Design review of the part shown in the three views and the two pictorial views. Dimensions are in mm from the part's minimum x, y and z. A direction names the side the tool comes from. Round coordinates to 2 decimals unless told otherwise and drop trailing zeros. Loops run counter-clockwise (first coordinate to the right, second up) from the corner with the lowest first, then second, coordinate; pieces in that order, holes last.
1. To check wall thickness, follow line 1 along Z through (x, y) = (34, 12.7); line 2 along X through (y, z) = (11.5, 7.5); line 3 along X through (y, z) = (11.25, 10.5). State the ranges of each line that lie inside material, in increasing order.
2. Draft analysis for pull direction X (two halves, no side actions). For the marked faces 4, 5 and 6, state which applies: released by +X, released by -X, zero draft, split by the parting line, or undercut.
3. Clearance check with flat-ended pins moving along their axes: pin 1 Ø12 at (y, z) = (12, 31.5) entering from -X; pin 2 Ø12 at (x, y) = (33, 3) entering from +Z; pin 3 Ø2 at (x, y) = (57.5, 4) entering from +Z. State where each tip first meets the part, or that it passes through.
4. Consider section D-D on x = 36. State the section outline as (y, z) points.
5. Consider section A-A on y = 13.5. State the section outline as (x, z) points, then the cut area to 3 significant figures.
6. Consider section C-C on x = 7.5. State the section outline as (y, z) points, then the cut area to 3 significant figures.
7. Tool access review of the marked faces 1, 2 and 3: name each direction out of +Z, -Z, +X, -X, +Y, -Y from which nothing blocks a thin tool from reaching the whole face with its end or side.
8. Consider section B-B on z = 30. State the section outline as (x, y) points, then the cut area to 3 significant figures.
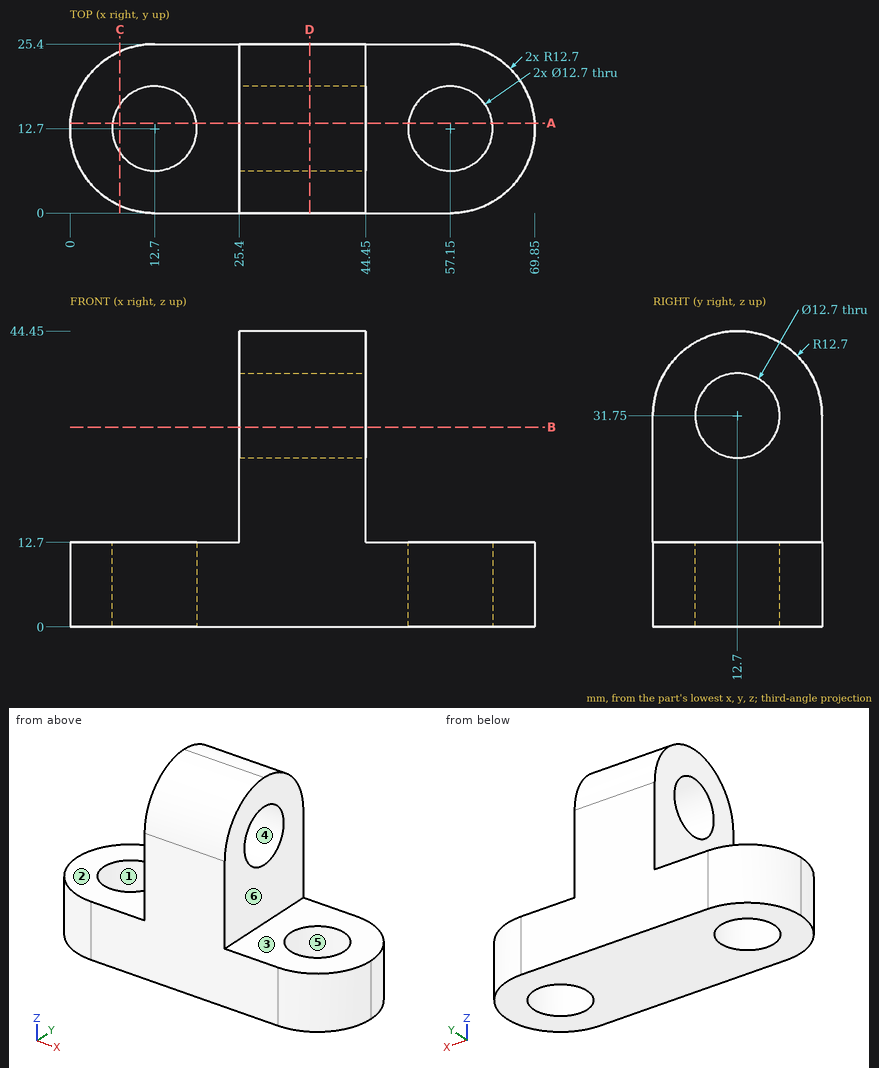
Resolved:
1. line 1: z = 0 to 25.4, 38.1 to 44.45
1. line 2: x = 0.06 to 6.46, 18.94 to 50.91, 63.39 to 69.79
1. line 3: x = 0.08 to 6.52, 18.88 to 50.97, 63.33 to 69.77
2. face 4: zero draft
2. face 5: undercut
2. face 6: released by +X
3. pin 1: stops at x = 25.4
3. pin 2: stops at z = 43.9
3. pin 3: stops at z = 12.7
4. outline: (0, 0) - (25.4, 0) - (25.4, 31.75) arc R12.7 ccw to (12.7, 44.45) arc R12.7 ccw to (0, 31.75) - close; hole circle Ø12.7 at (12.7, 31.75)
5. outline: (0.03, 0) - (6.4, 0) - (6.4, 12.7) - (0.03, 12.7) - close; (19, 0) - (50.85, 0) - (50.85, 12.7) - (44.45, 12.7) - (44.45, 25.45) - (25.4, 25.45) - (25.4, 12.7) - (19, 12.7) - close; (25.4, 38.05) - (44.45, 38.05) - (44.45, 44.42) - (25.4, 44.42) - close; (63.45, 0) - (69.82, 0) - (69.82, 12.7) - (63.45, 12.7) - close
5. area: 931 mm2
6. outline: (1.11, 0) - (9.06, 0) - (9.06, 12.7) - (1.11, 12.7) - close; (16.34, 0) - (24.29, 0) - (24.29, 12.7) - (16.34, 12.7) - close
6. area: 202 mm2
7. face 1: +Z, -Z
7. face 2: +Z, -X, +Y, -Y
7. face 3: +Z, +X, +Y, -Y
8. outline: (25.4, 0) - (44.45, 0) - (44.45, 6.6) - (25.4, 6.6) - close; (25.4, 18.8) - (44.45, 18.8) - (44.45, 25.4) - (25.4, 25.4) - close
8. area: 251 mm2
